Autodesk Inventor part; units mm, degrees
ref_plane "YZ Plane" through (0, 0, 0) normal (1, 0, 0) x (0, 1, 0)
ref_plane "XZ Plane" through (0, 0, 0) normal (0, 1, 0) x (-1, 0, 0)
ref_plane "XY Plane" through (0, 0, 0) normal (0, 0, 1) x (1, 0, 0)
sketch "Sketch1" plane through (0, 0, 0) normal (0, 1, 0) x (-1, 0, 0)
  line L0 (0, 0) -> (6, 0)
  line L1 (6, 0) -> (6, -6)
  line L2 (6, -6) -> (0, -6)
  line L3 (0, -6) -> (0, 0)
  circle A0 centre (3, -3) radius 1.75
  dimension "d0" = 6
  dimension "d1" = 6
  dimension "d2" = 3.5
extrude "Extrusion1" add sketch "Sketch1" along normal blind 1.5
sketch "Sketch2" plane through (0, 1.5, 0) normal (0, 1, 0) x (1, 0, 0)
  line L0 (0, 6) -> (-6, 6)
  line L1 (-6, 6) -> (-6, 0)
  line L2 (-6, 0) -> (0, 0)
  line L3 (0, 0) -> (0, 6)
  circle A0 centre (-3, 3) radius 1.75
  line L4 (-6, 0) -> (-9.4, 0)
  line L5 (-9.4, 0) -> (-9.4, 6)
  line L6 (-9.4, 6) -> (-6, 6)
  line L7 (-6, 6) -> (-6, 0)
  dimension "d5" = 3.4
extrude "Extrusion2" add sketch "Sketch2" along normal blind 1.5
properties part number "12Vnub"
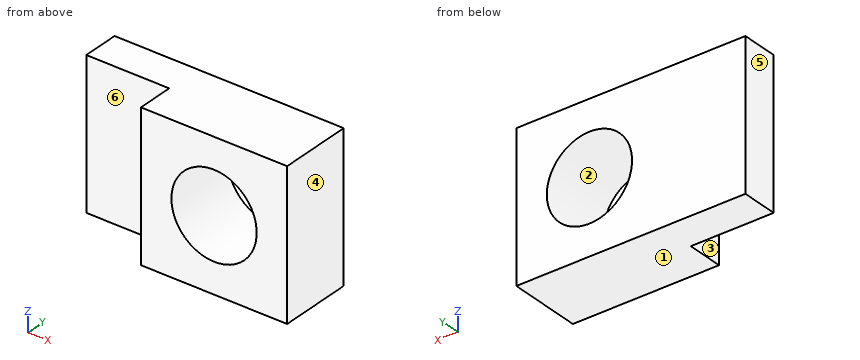
Can you work these out from the model? Positions are in its coordinate system, mm. Face numbers are marked on the shaded views. A direction names the side the tool comes from. Coordinates: 2 decimals unless noted, no trailing zeros. Write each loop counter-clockwise with the first axis right and the second up, starting at its lowest first coordinate (ties: lowest second). Pieces come first, ordered by that corner, then holes. Notation, with made-up numbers: (-10.5, 88) - (21.5, 88) arc R9 ccw to (21.5, 100) - close; hole circle Ø9 at (65.5, 61). An arc over 180 degrees is marked (long way). Return JSON: item names as keys, results as strings. Group by question number.
Item 1: Please list where these lines run through material, in increasing order: probe 1 along Z at (x, y) = (-3, 1.7); probe 2 along X at (y, z) = (1.8, -3).
Item 2: Which directions (+Z, -Z, +X, -X, +Y, -Y) give clear straight access to the entire face, cutting with the end or side of a thin tool? Please do the marked faces 5 and 6.
Item 3: If we section it at D-D (x = -7): Write out the boundary of the cut face in (y, z), then the cut area to 3 significant figures.
Item 4: I'm going to push flat-ended pins straight in: pin 1 Ø1.5 at (x, z) = (-7.5, -4.5) entering from -Y; pin 2 Ø1.6 at (y, z) = (0.5, -4) entering from -X. Where does each tip first touch, or does it pass through?
Item 5: If we section it at A-A (y = 1.4): Write out the boundary of the cut face in (x, z), then the cut area to 3 significant figures.
Item 6: We'd pull the mould along X, two halves only. Please class the marked faces 1, 2, 3 and 4: pulls with the +X half, pulls with the -X half, needs draft (parallel to the pull), parting line crosses it, or undercut.
Item 7: If we section it at C-C (y = 2.25): Write out the boundary of the cut face in (x, z).
Return value:
{
 "1": {"probe 1": "z = -6 to -4.75, -1.25 to 0", "probe 2": "x = -9.4 to -4.75, -1.25 to 0"},
 "2": {"face 5": "+Z, -Z, -X, +Y, -Y", "face 6": "+Z, -Z, -X, -Y"},
 "3": {"outline": "(1.5, -6) - (3, -6) - (3, 0) - (1.5, 0) - close", "area": "9.00 mm^2"},
 "4": {"pin 1": "stops at y = 1.5", "pin 2": "stops at x = -6"},
 "5": {"outline": "(-6, -6) - (0, -6) - (0, 0) - (-6, 0) - close; hole circle Ø3.5 at (-3, -3)", "area": "26.4 mm^2"},
 "6": {"face 1": "needs draft", "face 2": "undercut", "face 3": "pulls with the -X half", "face 4": "pulls with the +X half"},
 "7": {"outline": "(-9.4, -6) - (0, -6) - (0, 0) - (-9.4, 0) - close; hole circle Ø3.5 at (-3, -3)"}
}
